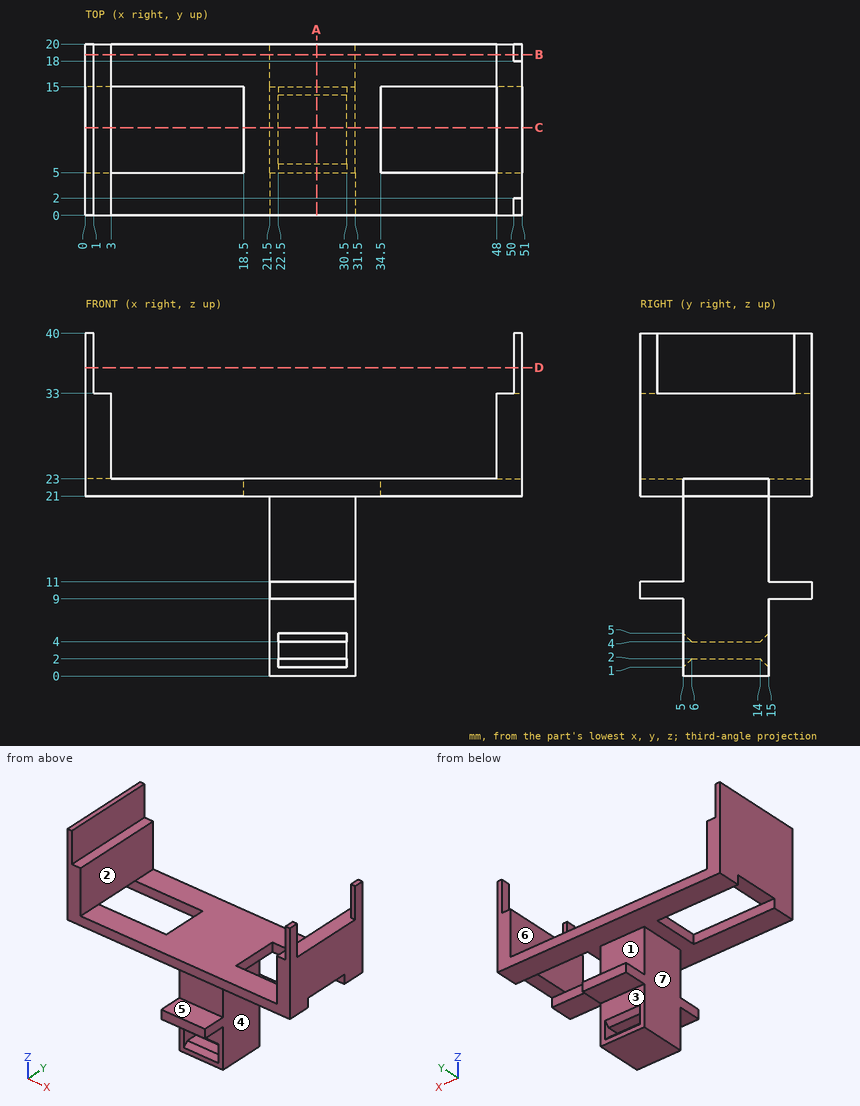
Study the drawing (mm; zero at the part's minimum x, y, z) and answer. A direction names the side the tool comes from. Coordinates: 2 decimals unless noted, no trailing zeros. Write each loop counter-clockwise with the first axis right and the second up, starting at its lowest first coordinate (ties: lowest second). Pieces come first, ordered by that corner, then holes. Notation, with made-up numbers: (7.25, 18.5) - (53.25, 18.5) arc R21 cw to (53.25, 31.5) - close; hole circle Ø6 at (89.25, -30). An arc over 180 degrees is marked (long way). One line per question, with ' | ' between items.
1) Consider probe 1 along X at (y, z) = (4, 32.5); probe 2 along Z at (x, y) = (24, 3); probe 3 along X at (y, z) = (1.25, 37.5). Determine where each line is inside the solid, lowest interval first. Write a range as [from, to].
Checks:
probe 1: [0, 3], [48, 51] | probe 2: [9, 11], [21, 23] | probe 3: [0, 1], [50, 51]
2) The mould has two halves that part along X. Classify the marked faces 5, 6 and 7: +X half, -X half, draft (parallel to the pull), parting line (faces both ways), or undercut.
Checks:
face 5: draft | face 6: undercut | face 7: -X half
3) Find section C-C, the plane y = 10.25. Determine the outline of the cut face in (x, z).
Checks:
outline: (0, 23) - (3, 23) - (3, 33) - (1, 33) - (1, 40) - (0, 40) - close; (18.5, 21) - (21.5, 21) - (21.5, 0) - (31.5, 0) - (31.5, 21) - (34.5, 21) - (34.5, 23) - (18.5, 23) - close; (48, 23) - (51, 23) - (51, 33) - (48, 33) - close; hole (22.5, 2) - (30.5, 2) - (30.5, 4) - (22.5, 4) - close
4) Find section B-B, the plane y = 18.75. Determine the outline of the cut face in (x, z).
Checks:
outline: (0, 21) - (51, 21) - (51, 40) - (50, 40) - (50, 33) - (48, 33) - (48, 23) - (3, 23) - (3, 33) - (1, 33) - (1, 40) - (0, 40) - close; (21.5, 9) - (31.5, 9) - (31.5, 11) - (21.5, 11) - close
5) For the marked faces 1, 2, 3 and 4, determine the directions among +Z, -Z, +X, -X, +Y, -Y from which every point of the face is accessible in a straight line to the end or side of a thin tool.
Checks:
face 1: +X, -X, +Y | face 2: +Z, +Y, -Y | face 3: -Z, +X, -X, +Y | face 4: -Z, +X, +Y, -Y
6) Flat-ended cylindrical pins translate along their axes: P1, Ø12, axis at x = 27.5, y = 16, coming from the +Z side; P2, Ø1.6, axis at y = 12, z = 22, coming from the -X side; P3, Ø1, axis at y = 8, z = 22, coming from the +X side. Find the tip coordinate at first contact, or state that the pin passes through.
Checks:
P1: z = 23 | P2: x = 18.5 | P3: x = 34.5
7) Find section D-D, the plane z = 36. Determine the outline of the cut face in (x, y).
Checks:
outline: (0, 0) - (1, 0) - (1, 20) - (0, 20) - close; (50, 0) - (51, 0) - (51, 2) - (50, 2) - close; (50, 18) - (51, 18) - (51, 20) - (50, 20) - close
8) Find section A-A, the plane x = 27. Determine the outline of the cut face in (y, z), and give its area (3 significant figures).
Checks:
outline: (0, 9) - (5, 9) - (5, 5) - (6, 4) - (14, 4) - (15, 5) - (15, 9) - (20, 9) - (20, 11) - (15, 11) - (15, 21) - (20, 21) - (20, 23) - (0, 23) - (0, 21) - (5, 21) - (5, 11) - (0, 11) - close; (5, 0) - (15, 0) - (15, 1) - (14, 2) - (6, 2) - (5, 1) - close | area: 248 mm2
